```python
from build123d import *

# Parameters (mm, degrees)
F1_DEPTH = 25
F3_W     = 25
F3_H     = 33
F3_H_2   = 17
F4_DEPTH = 5
F6_DEPTH = 25


# Not quite as in the source:
# - a fillet or chamfer that OpenCascade refuses, or shapes differently, is made with other operations: its cross-section is extruded or revolved along the edge and cut away or added


with BuildPart() as f1:
    # F0 (on Right) → F1 (new body)
    with BuildSketch(Plane.YZ):
        with BuildLine():
            ThreePointArc((0, 8), (5.6568542495, 5.6568542495), (8, 0))
            Line((8, 0), (12, 0))
            ThreePointArc((12, 0), (8.4852813742, 8.4852813742), (0, 12))
            Line((0, 12), (0, 8))
        make_face()
        with BuildLine():
            Line((12, 0), (8, 0))
            ThreePointArc((8, 0), (0, -8), (-8, 0))
            Line((-8, 0), (-12, 0))
            ThreePointArc((-12, 0), (0, -12), (12, 0))
        make_face()
        with BuildLine():
            ThreePointArc((-8, 0), (-5.6568542495, 5.6568542495), (0, 8))
            Line((0, 8), (0, 12))
            ThreePointArc((0, 12), (-8.4852813742, 8.4852813742), (-12, 0))
            Line((-12, 0), (-8, 0))
        make_face()
        with BuildLine():
            ThreePointArc((-12, 0), (-8.4852813742, 8.4852813742), (0, 12))
            Line((0, 12), (0, 25))
            Line((0, 25), (0, 29))
            Line((0, 29), (0, 33))
            Line((0, 33), (-12, 33))
            Line((-12, 33), (-12, 0))
        make_face()
        with BuildLine():
            ThreePointArc((0, 12), (8.4852813742, 8.4852813742), (12, 0))
            Line((12, 0), (12, 33))
            Line((12, 33), (0, 33))
            Line((0, 33), (0, 29))
            Line((0, 29), (0, 25))
            Line((0, 25), (0, 12))
        make_face()
    extrude(amount=F1_DEPTH)

    # F2: chamfer of 1 on 2 edges, made by hand

    # F2_s1 → F2_t2 (revolve, cut)
    with BuildSketch(Plane.XY):
        Polygon((24, -8), (25, -9), (25, -8), align=None)
    revolve(axis=Axis((25, 0, 0), (-1, 0, 0)), mode=Mode.SUBTRACT)

    # F2_s3 → F2_t4 (revolve, cut)
    with BuildSketch(Plane.XY):
        Polygon((1, -8), (0, -9), (0, -8), align=None)
    revolve(axis=Axis((0, 0, 0), (-1, 0, 0)), mode=Mode.SUBTRACT)

    # F3 (on face) → F4 (cut)
    with BuildSketch(Plane(origin=(0, 12, 0), x_dir=(-1, 0, 0), z_dir=(0, 1, 0))):
        with Locations((-12.5, 16.5)):
            Rectangle(F3_W, F3_H)
        with Locations((-12.5, -8.5)):
            Rectangle(F3_W, F3_H_2)
    extrude(amount=-F4_DEPTH, mode=Mode.SUBTRACT)

    # F5 (on face) → F6 (cut)
    with BuildSketch(Plane.XZ.offset(12)):
        with BuildLine():
            Line((12.5, 25), (8.5, 25))
            ThreePointArc((8.5, 25), (12.5, 21), (16.5, 25))
            Line((16.5, 25), (12.5, 25))
        make_face()
        with BuildLine():
            ThreePointArc((16.5, 25), (12.5, 29), (8.5, 25))
            Line((8.5, 25), (12.5, 25))
            Line((12.5, 25), (16.5, 25))
        make_face()
    extrude(amount=-F6_DEPTH, mode=Mode.SUBTRACT)


solid = f1.part
```
Source: CAD feature listing. Evaluate the final solid. Frame: model axes, mm. Give positions to 0.01 mm unless a question says otherwise; leave off trailing zeros. Order: outer loops, then holes, each group sorted by start corner. A loop starts at its lowest first (then second) coordinate and runs counter-clockwise, first axis right, second up.
(1) Section query D-D (x = 22). Return the cut outline in (y, z).
(2) Section query C-C (y = -10.25). Return the cut outline in (x, z), plus the area to 3 significant figures.
(3) Section query B-B (x = 12.5). Return the cut outline in (y, z), plus the area to 3 significant figures.
(4) Section query A-A (z = 25). Return the cut outline in (x, y).
(5) Material intervals for line 1 along Z through (x, y) = (12.5, -6.75); line 2 along Z through (x, y) = (12.5, 1.5); line 3 along X through (y, z) = (-7.25, 23), sorted ascending.
(6) Contact query for a flat-ended pin moving along its axis: P1, Ø5, axis at x = 8.5, y = -7.5, coming from the -Z side. Output: stop coordinate, or through.
(7) Pull-direction query (X, two-part tool) for faces 1 (the face through (11.979, -2.633, 28.966)), 2 (the face through (12.32, -5.64, -10.59)), 3 (the face through (0.826, -8.168, -0.302)); classes: +X half, -X half, draft (parallel to the pull), parting line (faces both ways), or undercut.
Outcome:
1. outline: (-12, 0) arc R12 ccw to (7, -9.75) - (7, -3.87) arc R8 cw (long way) to (7, 3.87) - (7, 33) - (-12, 33) - close
2. outline: (0, -6.24) - (25, -6.24) - (25, 33) - (0, 33) - close; hole circle Ø8 at (12.5, 25)
2. area: 931 mm2
3. outline: (-12, 0) arc R12 ccw to (7, -9.75) - (7, -3.87) arc R8 cw (long way) to (7, 3.87) - (7, 21) - (-12, 21) - close; (-12, 29) - (7, 29) - (7, 33) - (-12, 33) - close
3. area: 471 mm2
4. outline: (0, -12) - (8.5, -12) - (8.5, 7) - (0, 7) - close; (16.5, -12) - (25, -12) - (25, 7) - (16.5, 7) - close
5. line 1: z = -9.92 to -4.29, 4.29 to 21, 29 to 33
5. line 2: z = -11.91 to -7.86, 7.86 to 21, 29 to 33
5. line 3: x = 0 to 9.04, 15.96 to 25
6. P1: stops at z = -10.91
7. face 1: undercut
7. face 2: draft
7. face 3: -X half
